Here's the drawing with two shaded views (mm, measured from the low corner). I have some questions. Round coordinates to 2 decimals unless told otherwise and drop trailing zeros. Order: outer loops, then holes, each group sorted by start corner. A loop starts at its lowest first (then second) coordinate and runs counter-clockwise, first axis right, second up. Notation, with made-up numbers: M -12.75,36.25 L 24.25,36.25 A13 cw 24.25,53.25 Z; hole C 64,9.25 d3. An arc over 180 degrees is marked long. One line per question, with ' | ' between items.
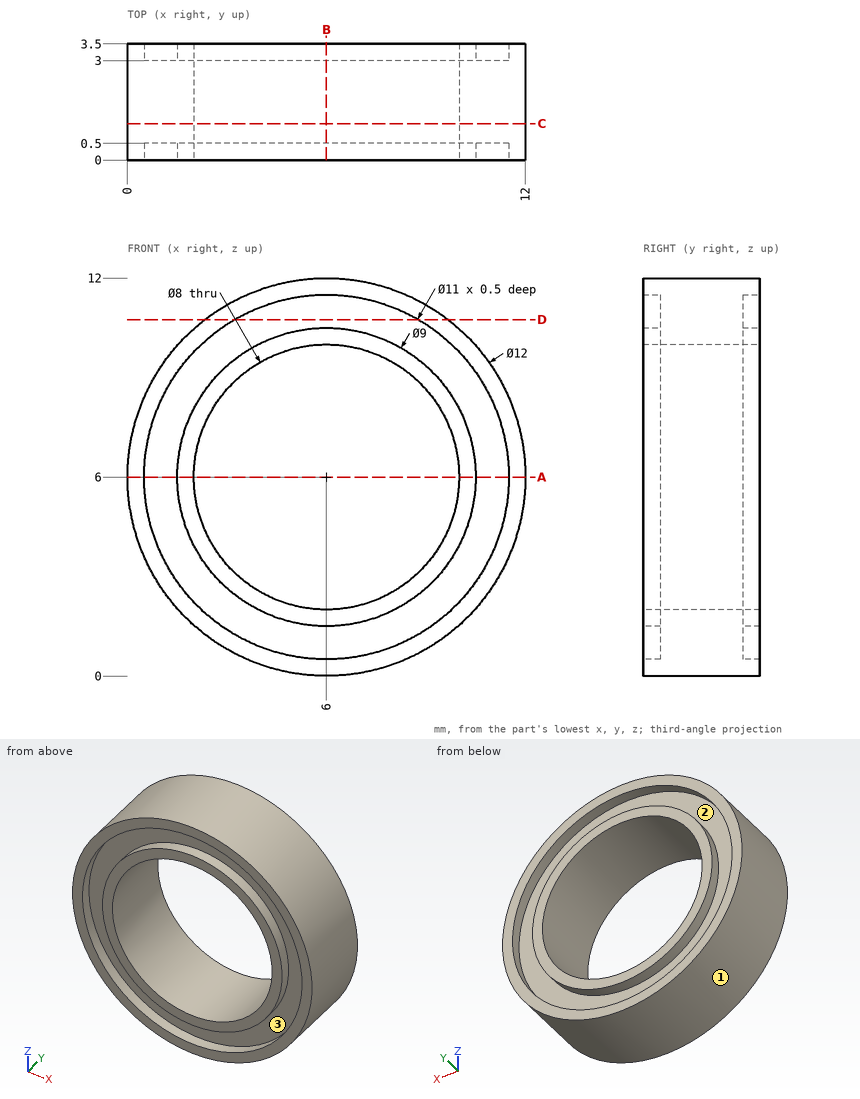
(1) If we section it at A-A on z = 6: Please give me the cut outline in (x, y).
Final values:
outline: M 0,0 L 0.5,0 L 0.5,0.5 L 1.5,0.5 L 1.5,0 L 2,0 L 2,3.5 L 1.5,3.5 L 1.5,3 L 0.5,3 L 0.5,3.5 L 0,3.5 Z; M 10,0 L 10.5,0 L 10.5,0.5 L 11.5,0.5 L 11.5,0 L 12,0 L 12,3.5 L 11.5,3.5 L 11.5,3 L 10.5,3 L 10.5,3.5 L 10,3.5 Z
(2) Will these pins go through, and if not, where does the flat tip stop? pin 1 Ø1.5 at (x, y) = (8, 1.5) entering from +Z; pin 2 Ø4 at (x, z) = (10.5, 7) entering from -Y; pin 3 Ø2 at (y, z) = (2.5, 4) entering from -X.
Final values:
pin 1: z = 11.87 | pin 2: y = 0 | pin 3: x = 0.08
(3) If we section it at C-C on y = 1.1: Please give me the cut outline in (x, z), plus the area to 3 significant figures.
Final values:
outline: C 6,6 d12; hole C 6,6 d8 | area: 62.8 mm^2
(4) Please list where these lines run through material, in increasing order: probe 1 along X at (y, z) = (0.2, 6); probe 2 along Z at (x, y) = (2.75, 3.05); probe 3 along Z at (x, y) = (3, 3.25). Write a range as [from, to].
Final values:
probe 1: [0, 0.5], [1.5, 2], [10, 10.5], [11.5, 12] | probe 2: [0.96, 1.56], [2.89, 3.67], [8.33, 9.11], [10.44, 11.04] | probe 3: [0.8, 1.39], [2.65, 3.35], [8.65, 9.35], [10.61, 11.2]
(5) If we section it at D-D on z = 10.75: Please give me the cut outline in (x, y).
Final values:
outline: M 2.33,0 L 3.23,0 L 3.23,0.5 L 8.77,0.5 L 8.77,0 L 9.67,0 L 9.67,3.5 L 8.77,3.5 L 8.77,3 L 3.23,3 L 3.23,3.5 L 2.33,3.5 Z
(6) Thinking about a two-plate mould opening in X: for the marked faces 1, 2 and 3, which applies, released by +X, released by -X, zero draft, split by the parting line, or undercut?
Final values:
face 1: split by the parting line | face 2: undercut | face 3: undercut
(7) If we section it at B-B on x = 6: Please give me the cut outline in (y, z).
Final values:
outline: M 0,0 L 3.5,0 L 3.5,0.5 L 3,0.5 L 3,1.5 L 3.5,1.5 L 3.5,2 L 0,2 L 0,1.5 L 0.5,1.5 L 0.5,0.5 L 0,0.5 Z; M 0,10 L 3.5,10 L 3.5,10.5 L 3,10.5 L 3,11.5 L 3.5,11.5 L 3.5,12 L 0,12 L 0,11.5 L 0.5,11.5 L 0.5,10.5 L 0,10.5 Z
